Here's how the part is built. I have some questions about the finished solid (model axes, mm). Coordinates: 2 decimals unless noted, no trailing zeros. Write each loop counter-clockwise with the first axis right and the second up, starting at its lowest first coordinate (ties: lowest second). Pieces come first, ordered by that corner, then holes. Notation, with made-up numbers: M -33.5,15.5 L -16.5,15.5 A12 ccw -16.5,37.5 Z; hole C 46.5,52.25 d3. An arc over 180 degrees is marked long. Use one line per item in the form item = value. Start each with the question number.
1. I want a section at D-D, the plane x = -45.5. List the corners of the cut face in (y, z) for me (1 decimal), plus the area to 3 significant figures.
2. Please list where these lines run through material, in increasing order: line 1 along Y through (x, z) = (0, -3) (3 decimals); line 2 along X through (y, z) = (-14, -2.8); line 3 along X through (y, z) = (-15.5, -3.2). Write a range as [from, to].
3. I want a section at C-C, the plane z = -2.55. List the corners of the cut face in (x, y) for me (1 decimal), plus the area to 3 significant figures.
4. I'm going to push a flat-ended pin straight in: pin 1 Ø7 at (x, y) = (0, -77.79) entering from -Z. Where does the tip first touch, or does it pass through?
5. I want a section at A-A, the plane x = 0. List the corners of the cut face in (y, z) for me (1 decimal), plus the area to 3 significant figures.
6. I want a section at B-B, the plane x = 64. List the corners of the cut face in (y, z) for me (1 decimal).
7. Thinking about a two-plate mould opening in Y: for faces 1 (the face through (41.092, -46.811, -2.348)), 2 (the face through (74.612, -4, -2)), 3 (the face through (1, 0, -2)), 4 (the face through (-0.519, -73.832, -2.348)), which applies, released by +Y, released by -Y, zero draft, split by the parting line, or undercut?
from build123d import *

# Parameters (mm, degrees)
F0_W     = 38.1
F0_H     = 92.075
F1_DEPTH = 4.7625
F3_DEPTH = 4.7625
F4_R     = 3.98907
F5_DEPTH = 4.7635


with BuildPart() as f1:
    # F0 (on Top) → F1 (new body)
    with BuildSketch(Plane.XY):
        with Locations((0, -46.0375)):
            Rectangle(F0_W, F0_H)
    extrude(amount=-F1_DEPTH)

    # F2 (on Top) → F3 (join)
    with BuildSketch(Plane.XY):
        with BuildLine():
            Line((-19.05, 0), (-74.6125, 0))
            Line((-74.6125, 0), (-74.6125, -8.212815))
            ThreePointArc((-74.6125, -8.212815), (-41.0845, -46.0375), (-74.6125, -83.862185))
            Line((-74.6125, -83.862185), (-74.6125, -92.075))
            Line((-74.6125, -92.075), (-19.05, -92.075))
            Line((-19.05, -92.075), (-19.05, 0))
        make_face()
        with BuildLine():
            Line((74.6125, -8.212815), (74.6125, 0))
            Line((74.6125, 0), (19.05, 0))
            Line((19.05, 0), (19.05, -92.075))
            Line((19.05, -92.075), (74.6125, -92.075))
            Line((74.6125, -92.075), (74.6125, -83.862185))
            ThreePointArc((74.6125, -83.862185), (41.0845, -46.0375), (74.6125, -8.212815))
        make_face()
    extrude(amount=-F3_DEPTH)

    # F4 (on Top) → F5 (cut, through all)
    with BuildSketch(Plane.XY):
        with Locations((0, -14.2875)):
            Circle(F4_R)
        with Locations((0, -77.7875)):
            Circle(F4_R)
    extrude(amount=-F5_DEPTH, mode=Mode.SUBTRACT)


solid = f1.part
Answer list:
q1.outline = M -92.1,-4.8 L -63.8,-4.8 L -63.8,0 L -92.1,0 Z; M -28.2,-4.8 L 0,-4.8 L 0,0 L -28.2,0 Z
q1.area = 269 mm²
q2.line_1 = [-92.075, -81.777], [-73.798, -18.277], [-10.298, 0]
q2.line_2 = [-58.56, -3.98], [3.98, 58.56]
q2.line_3 = [-56.4, -3.8], [3.8, 56.4]
q3.outline = M -74.6,-92.1 L 74.6,-92.1 L 74.6,-83.9 A38.1 cw 74.6,-8.2 L 74.6,0 L -74.6,0 L -74.6,-8.2 A38.1 cw -74.6,-83.9 Z; hole C 0,-77.8 d8; hole C 0,-14.3 d8
q3.area = 9,770 mm²
q4.pin_1 = through
q5.outline = M -92.1,-4.8 L -81.8,-4.8 L -81.8,0 L -92.1,0 Z; M -73.8,-4.8 L -18.3,-4.8 L -18.3,0 L -73.8,0 Z; M -10.3,-4.8 L 0,-4.8 L 0,0 L -10.3,0 Z
q5.area = 363 mm²
q6.outline = M -92.1,-4.8 L -81,-4.8 L -81,0 L -92.1,0 Z; M -11.1,-4.8 L 0,-4.8 L 0,0 L -11.1,0 Z
q7.face_1 = undercut
q7.face_2 = zero draft
q7.face_3 = released by +Y
q7.face_4 = undercut
